Part model, mm, in its own coordinate system. A direction names the side the tool comes from. Coordinates: 2 decimals unless noted, no trailing zeros. Order: outer loops, then holes, each group sorted by start corner. A loop starts at its lowest first (then second) coordinate and runs counter-clockwise, first axis right, second up. Notation, with made-up numbers: (23.5, -29) - (72.5, -29) arc R35 cw to (72.5, 7) - close; hole circle Ø11 at (38, -30.75). An arc over 180 degrees is marked (long way). Use a Markdown table: item, result. Add a question column.
1) Drop flat-ended pins along their axis: P1, Ø6, axis at y = 94, z = 5.5, coming from the +X side; P2, Ø2, axis at x = 36.5, z = 11, coming from the +Y side. Give the stop position or say it passes through.
2) Saw through at B-B on y = 105. List the corners of the cut face in (x, z).
3) Wall check: L1, parallel to Z at x = 22.5, y = 105; L2, parallel to Y at x = 11.5, z = 12; L3, parallel to X at y = 96, z = 3.75. Give the ranges that are in metal, low to high. Write a range as [from, to].
4) Saw through at C-C on x = 20.5. List the corners of the cut face in (y, z), then the cut area to 3 significant figures.
5) Saw through at D-D on x = 36.5. List the corners of the cut face in (y, z), then the cut area to 3 significant figures.
6) Tool access for faces 1 (the face through (17.5, 101, 6)), 2 (the face through (47.15, 3.01, 7.6)), 3 (the face through (32.5, 99, 7)): list every direction of +Z, -Z, +X, -X, +Y, -Y with a clear straight run to the whole face (end or side of a thin tool).
```python
from build123d import *

# Parameters (mm, degrees)
F1_DEPTH = 15
F2_R     = 7.49999
F3_R     = 10
F4_R     = 4
F5_DEPTH = 15


# Not quite as in the source:
# - a fillet or chamfer is up to 0.001 mm smaller than in the source, because OpenCascade refuses the exact size


with BuildPart() as f1:
    # F0 (on Top) → F1 (new body)
    with BuildSketch(Plane.XY):
        Polygon((0, 90), (0, 0), (50, 0), (50, 90), (32.5, 90), (32.5, 120), (17.5, 120), (17.5, 90), align=None)
    extrude(amount=F1_DEPTH)

    # F2 (radius 7.5 in the source; OpenCascade refuses exactly that, so slightly less here)
    f2_edges = [f1.edges().sort_by_distance(p)[0] for p in [
        (17.5, 120, 7.5),
        (32.5, 120, 7.5),
    ]]
    fillet(f2_edges, radius=F2_R)

    # F3
    f3_edges = [f1.edges().sort_by_distance(p)[0] for p in [
        (0, 90, 7.5),
        (50, 90, 7.5),
        (50, 0, 7.5),
        (0, 0, 7.5),
    ]]
    fillet(f3_edges, radius=F3_R)

    # F4 (on face) → F5 (cut)
    with BuildSketch(Plane.YZ.offset(32.5)):
        with Locations((105, 7.5)):
            Circle(F4_R)
    extrude(amount=-F5_DEPTH, mode=Mode.SUBTRACT)


solid = f1.part
```
Results are:
| question | item | result |
|---|---|---|
| 1 | P1 | x = 32.5 |
| 1 | P2 | y = 90 |
| 2 | outline | (17.5, 0) - (32.5, 0) - (32.5, 3.5) - (17.5, 3.5) - close; (17.5, 11.5) - (32.5, 11.5) - (32.5, 15) - (17.5, 15) - close |
| 3 | L1 | [0, 3.5], [11.5, 15] |
| 3 | L2 | [0, 90] |
| 3 | L3 | [17.5, 32.5] |
| 4 | outline | (0, 0) - (118.5, 0) - (118.5, 15) - (0, 15) - close; hole circle Ø8 at (105, 7.5) |
| 4 | area | 1,730 mm2 |
| 5 | outline | (0, 0) - (90, 0) - (90, 15) - (0, 15) - close |
| 5 | area | 1,350 mm2 |
| 6 | face 1 | +Z, -Z, -X, +Y |
| 6 | face 2 | +Z, -Z, +X, -Y |
| 6 | face 3 | +Z, -Z, +X, +Y |
